Could you check a few things on this model? Use its own coordinates, in mm. Round coordinates to 2 decimals unless told otherwise and drop trailing zeros. Write each loop counter-clockwise with the first axis right and the second up, starting at its lowest first coordinate (ties: lowest second). Pieces come first, ordered by that corner, then holes. Notation, with made-up numbers: (13.5, 63) - (68.5, 63) arc R23 ccw to (68.5, 79) - close; hole circle Ø6 at (18.5, 54). An arc over 180 degrees is marked (long way). Write each question's results on one line, items separated by ' | '. Start each with the question number.
(1) Imagine slicing it at A-A on z = -3.5. Write out the boundary of the cut face in (x, y), then the cut area to 3 significant figures.
(2) For P1, Ø2, axis at y = 4, z = -15, coming from the +X side; P2, Ø3, axis at x = 48.5, y = 3, coming from the -Z side; P3, Ø3, axis at y = 4, z = -8.5, coming from the -X side, each with a flat end and sliding along its axis, tell me the tip position at first contact or that it passes through.
(3) Imagine slicing it at C-C on y = 1.1. Write out the boundary of the cut face in (x, z).
(4) Please list where these lines run through material, in increasing order: line 1 (Z direction, x = 11, y = 3.4); line 2 (X direction, y = 3.2, z = 1.5); line 3 (Z direction, x = -50, y = 4.4). Write a range as [from, to].
(5) Imagine slicing it at B-B on x = 1. Write out the boundary of the cut face in (y, z).
(6) Imagine slicing it at D-D on x = -39.5. Write out the boundary of the cut face in (y, z).
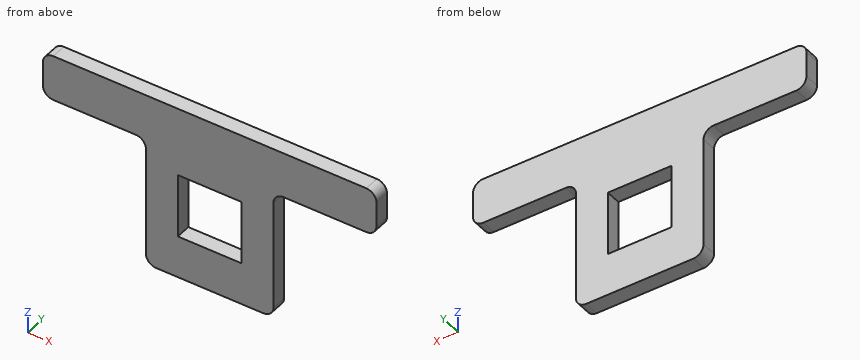
```python
from build123d import *

# Parameters (mm, degrees)
BOSS_EXTRUDE1_DEPTH = 6
FILLET1_R           = 4
SKETCH2_W           = 25
SKETCH2_H           = 25
CUT_EXTRUDE1_DEPTH  = 6


with BuildPart() as part:
    # Sketch1 → Boss-Extrude1 (new body)
    with BuildSketch(Plane(origin=(0, 0, 0), x_dir=(1, 0, 0), z_dir=(0, 1, 0))):
        Polygon((-65.35, -34.31), (65.35, -34.31), (65.35, -16.47), (25, -16.47), (25, 34.31), (-25, 34.31), (-25, -16.47), (-65.35, -16.47), align=None)
    extrude(amount=BOSS_EXTRUDE1_DEPTH)

    # Fillet1
    fillet1_edges = [part.edges().sort_by_distance(p)[0] for p in [
        (65.35, 3, 34.31),
        (-65.35, 3, 34.31),
        (-65.35, 3, 16.47),
        (-25, 3, 16.47),
        (-25, 3, -34.31),
        (25, 3, -34.31),
        (25, 3, 16.47),
        (65.35, 3, 16.47),
    ]]
    fillet(fillet1_edges, radius=FILLET1_R)

    # Sketch2 → Cut-Extrude1 (cut)
    with BuildSketch(Plane(origin=(0, 6, 0), x_dir=(1, 0, 0), z_dir=(0, 1, 0))):
        with Locations((0, 5.216940009)):
            Rectangle(SKETCH2_W, SKETCH2_H)
    extrude(amount=-CUT_EXTRUDE1_DEPTH, mode=Mode.SUBTRACT)


solid = part.part
```
Response:
1) outline: (-25, 0) - (-12.5, 0) - (-12.5, 6) - (-25, 6) - close; (12.5, 0) - (25, 0) - (25, 6) - (12.5, 6) - close | area: 150 mm²
2) P1: x = 25 | P2: z = 16.47 | P3: x = -25
3) outline: (-65.35, 20.47) arc R4 ccw to (-61.35, 16.47) - (-29, 16.47) arc R4 cw to (-25, 12.47) - (-25, -30.31) arc R4 ccw to (-21, -34.31) - (21, -34.31) arc R4 ccw to (25, -30.31) - (25, 12.47) arc R4 cw to (29, 16.47) - (61.35, 16.47) arc R4 ccw to (65.35, 20.47) - (65.35, 30.31) arc R4 ccw to (61.35, 34.31) - (-61.35, 34.31) arc R4 ccw to (-65.35, 30.31) - close; hole (-12.5, -17.72) - (12.5, -17.72) - (12.5, 7.28) - (-12.5, 7.28) - close
4) line 1: [-34.31, -17.72], [7.28, 34.31] | line 2: [-25, -12.5], [12.5, 25] | line 3: [16.47, 34.31]
5) outline: (0, -34.31) - (6, -34.31) - (6, -17.72) - (0, -17.72) - close; (0, 7.28) - (6, 7.28) - (6, 34.31) - (0, 34.31) - close
6) outline: (0, 16.47) - (6, 16.47) - (6, 34.31) - (0, 34.31) - close
